For this review, take the finished solid that the model builds, in its own axes (mm). Face numbers are marked on the shaded views. A direction names the side the tool comes from. Give positions to 0.01 mm unless a question says otherwise; leave off trailing zeros. Loops run counter-clockwise (first coordinate to the right, second up) from the corner with the lowest first, then second, coordinate; pieces in that order, holes last.
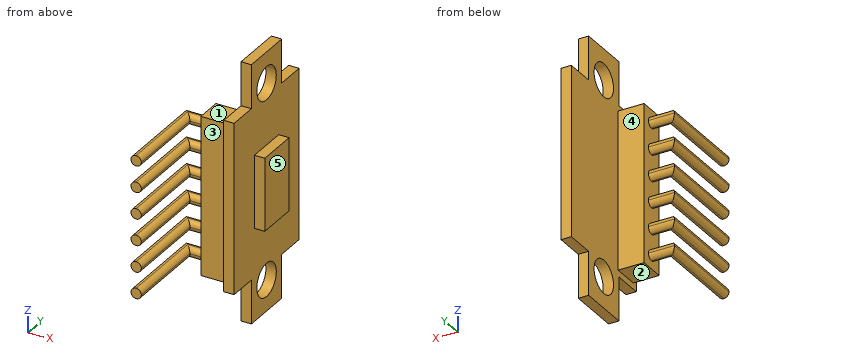
```python
from build123d import *

# Parameters (mm, degrees)
SKETCH1_R              = 1.6
BOSS_EXTRUDE1_DEPTH    = 1
SKETCH2_W              = 7
SKETCH2_H              = 4
BOSS_EXTRUDE2_DEPTH    = 1
SKETCH4_W              = 15.24
SKETCH4_H              = 2.5
BOSS_EXTRUDE3_DEPTH    = 2.5
SKETCH6_W              = 1
SKETCH6_H              = 1
BOSS_EXTRUDE4_DEPTH    = 2.5
SKETCH8_W              = 1
SKETCH8_H              = 1
BOSS_EXTRUDE5_DEPTH    = 8
FILLET1_R              = 0.5
LPATTERN1_COUNT        = 6
LPATTERN1_PITCH        = 2.54
FILLET1_OF_LPATTERN1_R = 0.5


with BuildPart() as part:
    # Sketch1 → Boss-Extrude1 (new body)
    with BuildSketch(Plane(origin=(0, 0, 0), x_dir=(0, 0, -1), z_dir=(1, 0, 0))):
        Polygon((-8.205, 2.5), (-12.415, 2.5), (-12.415, -2.5), (-8.205, -2.5), (-8.205, -5.35), (8.205, -5.35), (8.205, -2.5), (12.415, -2.5), (12.415, 2.5), (8.205, 2.5), (8.205, 5.35), (-8.205, 5.35), align=None)
        with Locations((-9.415, 0)):
            Circle(SKETCH1_R, mode=Mode.SUBTRACT)
        with Locations(Location((9.415, 0, 0), (0, 0, 180))):
            Circle(SKETCH1_R, mode=Mode.SUBTRACT)
    extrude(amount=BOSS_EXTRUDE1_DEPTH)

    # Sketch2 → Boss-Extrude2 (add)
    with BuildSketch(Plane(origin=(1, 0, 0), x_dir=(0, 0, -1), z_dir=(1, 0, 0))):
        Rectangle(SKETCH2_W, SKETCH2_H)
    extrude(amount=BOSS_EXTRUDE2_DEPTH)

    # Sketch4 → Boss-Extrude3 (add)
    with BuildSketch(Plane(origin=(0, 6.053191046, 0.231711856), x_dir=(0, 0, 1), z_dir=(-1, 0, 0))):
        with Locations((-0.231711856, -9.653191046)):
            Rectangle(SKETCH4_W, SKETCH4_H)
    extrude(amount=BOSS_EXTRUDE3_DEPTH)

    # Sketch6 → Boss-Extrude4 (add)
    with BuildSketch(Plane(origin=(-2.5, 6.053191046, 0.231711856), x_dir=(0, 0, 1), z_dir=(-1, 0, 0))):
        with Locations((-6.581711856, -9.633191046)):
            Rectangle(SKETCH6_W, SKETCH6_H)
    boss_extrude4 = extrude(amount=BOSS_EXTRUDE4_DEPTH)

    # Sketch8 → Boss-Extrude5 (add)
    with BuildSketch(Plane(origin=(1, -4.08, 0.231711856), x_dir=(0, 0, 1), z_dir=(0, -1, 0))):
        with Locations((-6.581711856, 5.5)):
            Rectangle(SKETCH8_W, SKETCH8_H)
    boss_extrude5 = extrude(amount=BOSS_EXTRUDE5_DEPTH)

    # Fillet1
    fillet1_edges = [part.edges().sort_by_distance(p)[0] for p in [
        (-4, -8.08, -5.85),
        (-4, -8.08, -6.85),
        (-3.25, -4.08, -5.85),
        (-3.25, -4.08, -6.85),
        (-3.75, -3.08, -5.85),
        (-3.75, -3.08, -6.85),
        (-5, -7.58, -5.85),
        (-5, -7.58, -6.85),
    ]]
    fillet(fillet1_edges, radius=FILLET1_R - 0.0001)  # a hair under: the kernel refuses the full size

    # LPattern1: Boss-Extrude4, Boss-Extrude5 ×6
    with Locations(*[(0, 0, i * LPATTERN1_PITCH) for i in range(1, LPATTERN1_COUNT)]):
        add(boss_extrude4)
        add(boss_extrude5)

    # Fillet1 of LPattern1
    fillet1_of_lpattern1_edges = [part.edges().sort_by_distance(p)[0] for p in [
        (-4, -8.08, -3.31),
        (-4, -8.08, -4.31),
        (-3.25, -4.08, -3.31),
        (-3.25, -4.08, -4.31),
        (-3.75, -3.08, -3.31),
        (-3.75, -3.08, -4.31),
        (-5, -7.58, -3.31),
        (-5, -7.58, -4.31),
        (-4, -8.08, -0.77),
        (-4, -8.08, -1.77),
        (-3.25, -4.08, -0.77),
        (-3.25, -4.08, -1.77),
        (-3.75, -3.08, -0.77),
        (-3.75, -3.08, -1.77),
        (-5, -7.58, -0.77),
        (-5, -7.58, -1.77),
        (-4, -8.08, 1.77),
        (-4, -8.08, 0.77),
        (-3.25, -4.08, 1.77),
        (-3.25, -4.08, 0.77),
        (-3.75, -3.08, 1.77),
        (-3.75, -3.08, 0.77),
        (-5, -7.58, 1.77),
        (-5, -7.58, 0.77),
        (-4, -8.08, 4.31),
        (-4, -8.08, 3.31),
        (-3.25, -4.08, 4.31),
        (-3.25, -4.08, 3.31),
        (-3.75, -3.08, 4.31),
        (-3.75, -3.08, 3.31),
        (-5, -7.58, 4.31),
        (-5, -7.58, 3.31),
        (-4, -8.08, 6.85),
        (-4, -8.08, 5.85),
        (-3.25, -4.08, 6.85),
        (-3.25, -4.08, 5.85),
        (-3.75, -3.08, 6.85),
        (-3.75, -3.08, 5.85),
        (-5, -7.58, 6.85),
        (-5, -7.58, 5.85),
    ]]
    fillet(fillet1_of_lpattern1_edges, radius=FILLET1_OF_LPATTERN1_R - 0.0001)  # a hair under: the kernel refuses the full size


solid = part.part
```
Item 1: For L1, parallel to Y at x = 1.5, z = 3.25; L2, parallel to X at y = -1.5, z = -0.25; L3, parallel to Y at x = -1.5, z = -1, list the stretches that pass through material, from the lowest coordinate up.
Answer:
L1: y = -2 to 2
L2: x = 0 to 2
L3: y = -4.85 to -2.35
Item 2: The part is to be moulded in two halves that separate along X. For the marked faces 3, 4 and 5, say which applies: released by +X, released by -X, zero draft, split by the parting line, or undercut.
Answer:
face 3: undercut
face 4: zero draft
face 5: released by +X
Item 3: Clearance check with flat-ended pins moving along their axes: pin 1 Ø0.8 at (x, z) = (0.5, 10) entering from +Y; pin 2 Ø1.2 at (x, z) = (-1.5, -3) entering from +Y; pin 3 Ø2 at (x, y) = (-3.5, -7) entering from -Z; pin 4 Ø0.6 at (x, y) = (-3.5, -5.5) entering from +Z. State where each tip first meets the part, or that it passes through.
Answer:
pin 1: stops at y = 2.5
pin 2: stops at y = -2.35
pin 3: stops at z = -6.85
pin 4: passes through
Item 4: Tool access review of the marked faces 1 and 2: name each direction out of +Z, -Z, +X, -X, +Y, -Y from which nothing blocks a thin tool from reaching the whole face with its end or side.
Answer:
face 1: +Z, -X, +Y, -Y
face 2: -Z, -X, +Y, -Y
Item 5: Take a section at D-D on x = -3. State how many separate pieces and enclosed holes the cut face has, and give its area (3 significant figures).
Answer:
separate pieces: 6
enclosed holes: 0
area: 4.71 mm2
Item 6: Take a section at A-A on y = -0.5. Give the boundary of the cut face in (x, z) (3 decimals).
Answer:
outline: (0, -12.415) - (1, -12.415) - (1, -10.935) - (0, -10.935) - close; (0, -7.895) - (1, -7.895) - (1, -3.5) - (2, -3.5) - (2, 3.5) - (1, 3.5) - (1, 7.895) - (0, 7.895) - close; (0, 10.935) - (1, 10.935) - (1, 12.415) - (0, 12.415) - close
Item 7: Take a section at C-C on z = 5.25. Give the boundary of the cut face in (x, y).
Answer:
outline: (-2.5, -4.85) - (0, -4.85) - (0, -5.35) - (1, -5.35) - (1, 5.35) - (0, 5.35) - (0, -2.35) - (-2.5, -2.35) - close
Item 8: Take a section at B-B on x = 0.5. Give the boundary of the cut face in (y, z) (3 decimals).
Answer:
outline: (-5.35, -8.205) - (-2.5, -8.205) - (-2.5, -12.415) - (2.5, -12.415) - (2.5, -8.205) - (5.35, -8.205) - (5.35, 8.205) - (2.5, 8.205) - (2.5, 12.415) - (-2.5, 12.415) - (-2.5, 8.205) - (-5.35, 8.205) - close; hole circle Ø3.2 at (0, -9.415); hole circle Ø3.2 at (0, 9.415)
